For this review, take the finished solid that the model builds, in its own axes (mm). A direction names the side the tool comes from. Coordinates: 2 decimals unless noted, no trailing zeros. Loops run counter-clockwise (first coordinate to the right, second up) from the corner with the lowest first, then second, coordinate; pieces in that order, holes last. Notation, with made-up numbers: (-3, 57.5) -> (39, 57.5) arc R33 cw to (39, 92.5) -> close; hole circle Ø7 at (-20.75, 21.5). An arc over 180 degrees is marked (long way). Answer in a Markdown table with one row per item.
from build123d import *

# Parameters (mm, degrees)
SKETCH2_R           = 15
BOSS_EXTRUDE1_DEPTH = 180
SKETCH3_R           = 4
BOSS_EXTRUDE2_DEPTH = 36


with BuildPart() as part:
    # Sketch2 → Boss-Extrude1 (new body)
    with BuildSketch(Plane(origin=(0, 0, 0), x_dir=(0, 0, -1), z_dir=(1, 0, 0))):
        with Locations(Location((0, 0, 0), (0, 0, 180))):
            Circle(SKETCH2_R)
    boss_extrude1 = extrude(amount=BOSS_EXTRUDE1_DEPTH)

    # Sketch3 → Boss-Extrude2 (add)
    with BuildSketch(Plane(origin=(180, 0, 0), x_dir=(0, 0, -1), z_dir=(1, 0, 0))):
        Circle(SKETCH3_R)
    boss_extrude2 = extrude(amount=BOSS_EXTRUDE2_DEPTH)

    # Mirror1: Boss-Extrude1, Boss-Extrude2 across plane
    add(boss_extrude1.mirror(Plane(origin=(0, 0, 0), x_dir=(0, 0, 1), z_dir=(1, 0, 0))))
    add(boss_extrude2.mirror(Plane(origin=(0, 0, 0), x_dir=(0, 0, 1), z_dir=(1, 0, 0))))


solid = part.part
Item 1: Insertion check: pin 1 (10 mm diameter, centred on y = -10, z = -2.5, fed in from +X); pin 2 (10 mm diameter, centred on x = -136.5, z = -6, fed in from -Y); pin 3 (5 mm diameter, centred on x = 2, z = 6.5, fed in from -Y). Each pin has a flat end and moves straight along its axis. Give the tip position at first contact, or say it passes through.
Worked answers:
| item | result |
|---|---|
| pin 1 | x = 180 |
| pin 2 | y = -14.97 |
| pin 3 | y = -14.46 |
Item 2: Take a section at A-A, the plane y = 0. State the section outline as (x, z) points.
Worked answers:
| item | result |
|---|---|
| outline | (-216, -4) -> (-180, -4) -> (-180, -15) -> (180, -15) -> (180, -4) -> (216, -4) -> (216, 4) -> (180, 4) -> (180, 15) -> (-180, 15) -> (-180, 4) -> (-216, 4) -> close |
Item 3: For L1, parallel to X at y = 1.5, z = -8.25; L2, parallel to Z at x = -89, y = -1.25; L3, parallel to Z at x = -131, y = 1, list the stretches that pass through material, from the lowest coordinate up.
Worked answers:
| item | result |
|---|---|
| L1 | -180 to 180 |
| L2 | -14.95 to 14.95 |
| L3 | -14.97 to 14.97 |
Item 4: Take a section at C-C, the plane x = 33. State the section outline as (y, z) points, and give its area (3 significant figures).
Worked answers:
| item | result |
|---|---|
| outline | circle Ø30 at (0, 0) |
| area | 707 mm² |
Item 5: For faces 1 (the cylindrical face through (-197.748, -3.905, 0.867)), 2 (the flat face through (216, 0, 0)), 3 (the flat face through (180, 3, 3)), list the 3-axis set-ups (+Z, -Z, +X, -X, +Y, -Y) from which the entire face can be reached by the end or side of a thin tool; tool diameter is ignored.
Worked answers:
| item | result |
|---|---|
| face 1 | -X |
| face 2 | +Z, -Z, +X, +Y, -Y |
| face 3 | +X |
